Here's the drawing with two shaded views (mm, measured from the low corner). I have some questions. A direction names the side the tool comes from. Give positions to 0.01 mm unless a question says otherwise; leave off trailing zeros. Use a Markdown table: item, result. Add a question column.
1) Suppose I cut it at A-A on x = 6.35. Count the separate pieces of the cut face and the enclosed holes in it.
2) Which directions (+Z, -Z, +X, -X, +Y, -Y) give clear straight access to the entire face, cutting with the end or side of a thin tool? Please do the marked faces 1, 2, 3, 4 and 5.
3) We'd pull the mould along Y, two halves only. Please class the marked faces 6, 7, 8 and 9: +Y half, -Y half, draft (parallel to the pull), parting line (faces both ways), or undercut.
4) If I drill on line 1 along Z through (x, y) = (8.5, 5) (1 decimal); line 2 along X through (y, z) = (21.25, 27) (1 decimal); line 3 along X through (y, z) = (1, 3), over which ranges is the centre line in solid material (lowest first)? Write a range as [from, to].
5) Will these pins go through, and if not, where does the flat tip stop? pin 1 Ø2.5 at (x, z) = (26, 2) entering from +Y (1 decimal); pin 2 Ø4 at (x, y) = (5, 9) entering from +Z (1 decimal).
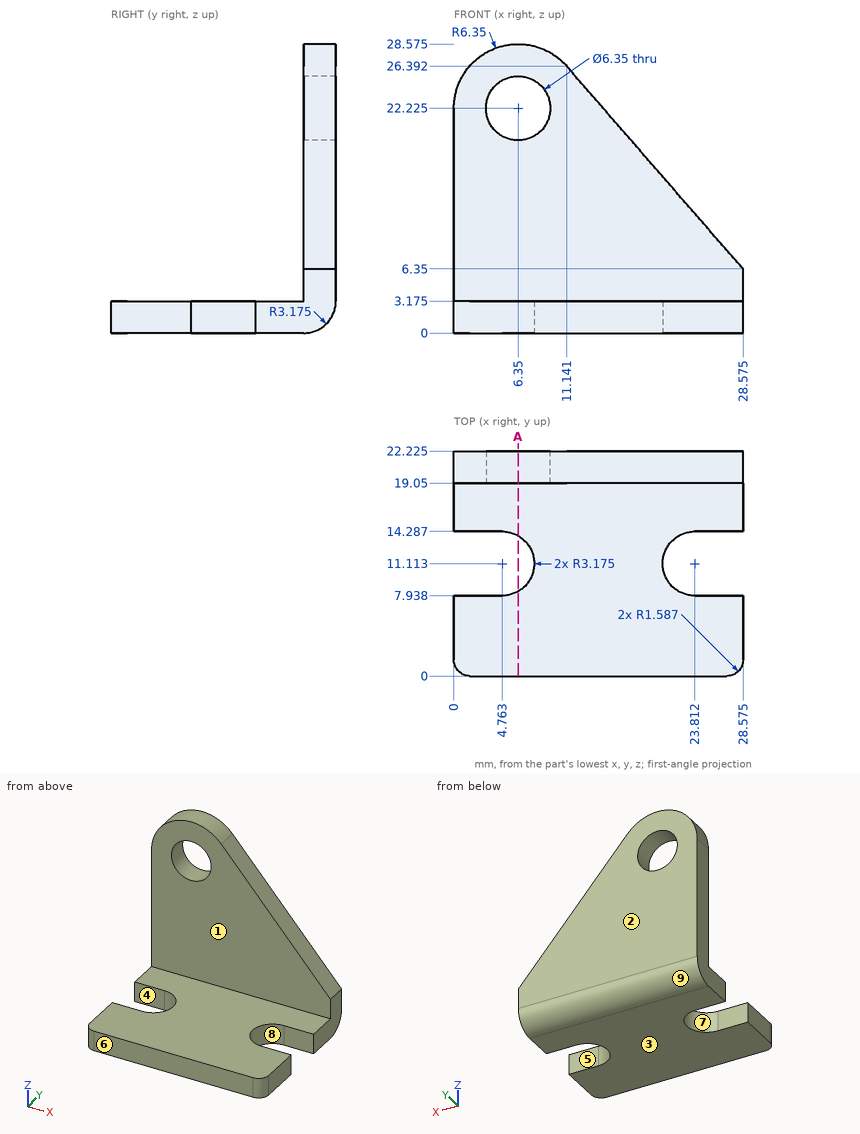
Answer block:
| question | item | result |
|---|---|---|
| 1 | separate pieces | 3 |
| 1 | enclosed holes | 0 |
| 2 | face 1 | +Z, +X, -X, -Y |
| 2 | face 2 | +Z, -Z, +X, -X, +Y |
| 2 | face 3 | -Z, +X, -X, +Y, -Y |
| 2 | face 4 | +Z, -Z, -X |
| 2 | face 5 | +Z, -Z, +X |
| 3 | face 6 | -Y half |
| 3 | face 7 | undercut |
| 3 | face 8 | undercut |
| 3 | face 9 | +Y half |
| 4 | line 1 | z = [0, 3.2] |
| 4 | line 2 | x = [2.2, 10.5] |
| 4 | line 3 | x = [0.11, 28.46] |
| 5 | pin 1 | stops at y = 22.2 |
| 5 | pin 2 | stops at z = 3.2 |
